Work out the finished part from the listing and answer in its coordinate system (mm). Face numbers are marked on the shaded views. A direction names the side the tool comes from. Round coordinates to 2 decimals unless told otherwise and drop trailing zeros. Write each loop counter-clockwise with the first axis right and the second up, starting at its lowest first coordinate (ties: lowest second). Pieces come first, ordered by that corner, then holes.
Autodesk Inventor part; units mm, degrees
ref_plane "Work Plane1" through (-56.3599, 0, 22) normal (0, 0, -1) x (-1, 0, 0)
ref_plane "YZ Plane" through (0, 0, 0) normal (1, 0, 0) x (0, 1, 0)
ref_plane "XZ Plane" through (0, 0, 0) normal (0, 1, 0) x (-1, 0, 0)
ref_plane "Work Plane1" through (-56.3599, 0, 22) normal (0, 0, -1) x (-1, 0, 0)
sketch "Sketch1" plane through (-56.3599, 0, 22) normal (0, 0, -1) x (-1, 0, 0)
  line L0 (-4.0299, -0.3538) -> (-2.2322, 1.4439) construction
  arc A0 (-1.4439, 2.2322) -> (-2.2322, 1.4439) centre (-0.9299, 0.9299) ccw construction
  line L1 (-1.4439, 2.2322) -> (0.3538, 4.0299) construction
  line L2 (-37.8299, 42.8299) -> (-37.8299, 37.8299) construction
  line L3 (-37.8299, 37.8299) -> (-42.9208, 37.8299) construction
  line L4 (-37.8299, 42.2137) -> (-37.8299, 45.8299) construction
  line L5 (-37.8299, 45.8299) -> (-4.0299, 45.8299) construction
  line L6 (-4.0299, 45.8299) -> (-4.0299, 42.2137) construction
  line L7 (-4.0299, 4.0299) -> (0.3538, 4.0299)
  circle A1 centre (-20.9299, 20.9299) radius 17.5
  line L8 (-20.9299, 58.9723) -> (17.1124, 20.9299) construction
  line L9 (17.1124, 20.9299) -> (-20.9299, -17.1124) construction
  line L10 (-20.9299, -17.1124) -> (-58.9723, 20.9299) construction
  line L11 (-58.9723, 20.9299) -> (-20.9299, 58.9723) construction
  line L12 (-20.9299, 58.9723) -> (-20.9299, -17.1124) construction
  line L13 (17.1124, 20.9299) -> (-58.9723, 20.9299) construction
  line L14 (-20.9299, 58.9723) -> (32.8701, 58.9723) construction
  line L15 (-43.4299, 43.4299) -> (1.5701, 43.4299) construction
  line L16 (1.5701, 43.4299) -> (1.5701, -1.5701) construction
  line L17 (1.5701, -1.5701) -> (-43.4299, -1.5701) construction
  line L18 (-43.4299, -1.5701) -> (-43.4299, 43.4299) construction
  line L19 (-43.4299, 43.4299) -> (1.5701, -1.5701) construction
  line L20 (1.5701, 43.4299) -> (-43.4299, -1.5701) construction
  line L21 (-43.4299, 5.3876) -> (-43.4299, 36.4723)
  line L22 (-43.4299, 36.4723) -> (-36.4723, 43.4299)
  line L23 (-36.4723, 43.4299) -> (-5.3876, 43.4299)
  line L24 (-5.3876, 43.4299) -> (1.5701, 36.4723)
  line L25 (1.5701, 36.4723) -> (1.5701, 5.3876)
  line L26 (1.5701, 5.3876) -> (-5.3876, -1.5701)
  line L27 (-5.3876, -1.5701) -> (-36.4723, -1.5701)
  line L28 (-36.4723, -1.5701) -> (-43.4299, 5.3876)
  line L29 (-4.0299, 42.2137) -> (-37.8299, 42.2137)
  line L30 (-4.0299, -0.3538) -> (-4.0299, 4.0299)
  circle A2 centre (-20.9299, 20.9299) radius 1.5
  line L31 (-10.9299, 10.9299) -> (-30.9299, 10.9299) construction
  line L32 (-30.9299, 10.9299) -> (-30.9299, 30.9299) construction
  line L33 (-30.9299, 30.9299) -> (-10.9299, 30.9299) construction
  line L34 (-10.9299, 30.9299) -> (-10.9299, 10.9299) construction
  line L35 (-10.9299, 10.9299) -> (-30.9299, 30.9299) construction
  line L36 (-30.9299, 10.9299) -> (-10.9299, 30.9299) construction
  circle A3 centre (-30.9299, 30.9299) radius 1.4
  circle A4 centre (-30.9299, 10.9299) radius 1.4
  circle A5 centre (-10.9299, 10.9299) radius 1.4
  line L37 (-45.8299, 37.8299) -> (-42.0723, 37.8299) construction
  line L38 (-42.1723, 37.7299) -> (-45.8299, 37.7299)
  line L39 (-45.8299, 37.7299) -> (-45.8299, 4.1299)
  line L40 (-45.8299, 4.1299) -> (-42.1723, 4.1299)
  line L41 (-42.1723, 4.1299) -> (-42.1723, 37.7299)
  line L42 (-45.8299, 4.0299) -> (-42.0723, 4.0299) construction
  line L43 (-45.8299, 37.8299) -> (-42.0723, 37.8299)
  line L44 (-37.7299, 45.8299) -> (-4.1299, 45.8299)
  line L45 (-4.1299, 45.8299) -> (-4.1299, 42.1723)
  line L46 (-4.1299, 42.1723) -> (-37.7299, 42.1723)
  line L47 (-37.7299, 42.1723) -> (-37.7299, 45.8299)
  line L48 (0.4701, 37.8299) -> (0.4701, 4.0299) construction
  line L49 (0.4701, 4.0299) -> (3.9701, 4.0299) construction
  line L50 (3.9701, 37.8299) -> (3.9701, 4.0299) construction
  line L51 (0.4701, 37.8299) -> (3.9701, 37.8299) construction
  line L52 (-45.8299, -3.9701) -> (-4.0299, -3.9701) construction
  line L53 (0.3124, 37.7299) -> (3.9701, 37.7299)
  line L54 (3.9701, 37.7299) -> (3.9701, 4.1299)
  line L55 (3.9701, 4.1299) -> (0.3124, 4.1299)
  line L56 (0.3124, 4.1299) -> (0.3124, 37.7299)
  line L57 (-4.1713, -0.3538) -> (-37.7299, -0.3538)
  line L58 (-37.7299, -0.3538) -> (-37.7299, -3.9701)
  line L59 (-37.7299, -3.9701) -> (-4.1713, -3.9701)
  line L60 (-4.1713, -3.9701) -> (-4.1713, -0.3538)
  point P0 (-37.8299, 4.0299)
  dimension "d18" = 53.8
  dimension "d19" = 45
  dimension "d20" = 53.8
  dimension "d21" = 45
  dimension "d22" = 45
  dimension "d30" = 20
  dimension "d31" = 20
  dimension "d32" = 2.8
  dimension "d33" = 2.8
  dimension "d34" = 2.8
  dimension "d35" = 3
  dimension "d36" = 0.1
  dimension "d37" = 0.1
  dimension "d38" = 0.1
  dimension "d39" = 0.1
extrude "Extrusion1" add sketch "Sketch1" along normal blind 6 contours L30 L26 L57 L28 L41 L22 L46 L24 L56 L7 | L7 L26 L30 | L56 L24 L25 L26 | L26 L25 L24 L53 L54 L55 | L60 L59 L58 L57 L28 L27 L26 | L26 L27 L28 L57 | L46 L22 L29 L24 | L24 L29 L45 | L40 L39 L38 L22 L21 L28 | L28 L21 L22 L41 | L29 L22 L23 L24 | L24 L23 L22 L29 L47 L44 L45 | L47 L29 L22 | A1 | A2 | A3 | A4 | A5
sketch "Skizze4" plane through (-56.3599, 0, 16) normal (0, 0, -1) x (-1, 0, 0)
  line L0 (-37.7299, 42.1723) -> (-42.1723, 37.7299)
  line L1 (-42.1723, 37.7299) -> (-45.8299, 37.7299)
  line L2 (-45.8299, 37.7299) -> (-45.8299, 4.1299) construction
  line L3 (-45.8299, 4.1299) -> (-42.1723, 4.1299)
  line L4 (-42.1723, 4.1299) -> (-37.6885, -0.3538)
  line L5 (-37.6885, -0.3538) -> (-37.7299, -0.3538)
  line L6 (-37.7299, -0.3538) -> (-37.7299, -3.9701)
  line L7 (-37.7299, -3.9701) -> (-4.1713, -3.9701) construction
  line L8 (-4.1713, -3.9701) -> (-4.1713, -0.3538)
  line L9 (-4.1713, -0.3538) -> (0.3124, 4.1299)
  line L10 (0.3124, 4.1299) -> (3.9701, 4.1299)
  line L11 (3.9701, 4.1299) -> (3.9701, 37.7299) construction
  line L12 (3.9701, 37.7299) -> (0.3124, 37.7299)
  line L13 (0.3124, 37.7299) -> (-4.1299, 42.1723)
  line L14 (-4.1299, 42.1723) -> (-4.1299, 45.8299)
  line L15 (-4.1299, 45.8299) -> (-37.7299, 45.8299) construction
  line L16 (-37.7299, 45.8299) -> (-37.7299, 42.1723)
  line L17 (-37.9299, 46.0299) -> (-3.9299, 46.0299) construction
  line L18 (-3.9299, 46.0299) -> (-3.9299, 42.2551)
  line L19 (-3.9299, 42.2551) -> (0.3953, 37.9299)
  line L20 (0.3953, 37.9299) -> (4.1701, 37.9299)
  line L21 (4.1701, 37.9299) -> (4.1701, 3.9299) construction
  line L22 (4.1701, 3.9299) -> (0.3953, 3.9299)
  line L23 (0.3953, 3.9299) -> (-3.9713, -0.4367)
  line L24 (-3.9713, -0.4367) -> (-3.9713, -4.1701)
  line L25 (-3.9713, -4.1701) -> (-37.9299, -4.1701) construction
  line L26 (-37.9299, -4.1701) -> (-37.9299, -0.3953)
  line L27 (-37.9299, -0.3953) -> (-42.2551, 3.9299)
  line L28 (-42.2551, 3.9299) -> (-46.0299, 3.9299)
  line L29 (-46.0299, 3.9299) -> (-46.0299, 37.9299) construction
  line L30 (-46.0299, 37.9299) -> (-42.2551, 37.9299)
  line L31 (-42.2551, 37.9299) -> (-37.9299, 42.2551)
  line L32 (-37.9299, 42.2551) -> (-37.9299, 46.0299)
  line L33 (-45.8299, 37.7299) -> (-45.8299, 37.9299)
  line L34 (-4.1299, 45.8299) -> (-37.7299, 45.8299)
  line L35 (-37.7299, 45.8299) -> (-37.9299, 45.8299)
  line L36 (-4.1299, 45.8299) -> (-3.9299, 45.8299)
  line L37 (3.9701, 37.7299) -> (3.9701, 37.9299)
  line L38 (3.9701, 4.1299) -> (3.9701, 37.7299)
  line L39 (3.9701, 4.1299) -> (3.9701, 3.9299)
  line L40 (-4.1713, -3.9701) -> (-3.9713, -3.9701)
  line L41 (-37.7299, -3.9701) -> (-37.9299, -3.9701)
  line L42 (-45.8299, 4.1299) -> (-45.8299, 3.9299)
  point P0 (-56.3599, 0)
  dimension "d40" = 0.2
extrude "IM_offset" add sketch "Skizze4" against normal up to surface (6 mm away)
ref_plane "Arbeitsebene5" through (-35.4299, 3.9299, 22) normal (-1, 0, 0) x (0, 0, 1)
ref_plane "Arbeitsebene6" through (-18.4299, 20.9299, 22) normal (0, 1, 0) x (-1, 0, 0)
sketch "Skizze31" plane through (-56.3599, 0, 16) normal (0, 0, -1) x (-1, 0, 0)
  line L0 (3.9701, 3.9299) -> (3.9701, 37.9299)
  line L1 (3.9701, 37.9299) -> (0.3953, 37.9299)
  line L2 (0.3953, 37.9299) -> (-3.9299, 42.2551)
  line L3 (-3.9299, 42.2551) -> (-3.9299, 45.8299)
  line L4 (-3.9299, 45.8299) -> (-37.9299, 45.8299)
  line L5 (-37.9299, 45.8299) -> (-37.9299, 42.2551)
  line L6 (-37.9299, 42.2551) -> (-42.2551, 37.9299)
  line L7 (-42.2551, 37.9299) -> (-45.8299, 37.9299)
  line L8 (-45.8299, 37.9299) -> (-45.8299, 3.9299)
  line L9 (-42.2551, 3.9299) -> (-45.8299, 3.9299)
  line L10 (-37.9299, -0.3953) -> (-42.2551, 3.9299)
  line L11 (-37.9299, -3.9701) -> (-37.9299, -0.3953)
  line L12 (-3.9713, -3.9701) -> (-37.9299, -3.9701)
  line L13 (-3.9713, -3.9701) -> (-3.9713, -0.4367)
  line L14 (-3.9713, -0.4367) -> (0.3953, 3.9299)
  line L15 (0.3953, 3.9299) -> (3.9701, 3.9299)
  circle A0 centre (-20.9506, 20.9092) radius 10
  point P0 (-56.3599, 0)
  dimension "d181" = 20
extrude "Extrusion26" cut sketch "Skizze31" against normal blind 10 contours A0
sketch "Skizze32" plane through (-56.3599, 0, 16) normal (0, 0, -1) x (-1, 0, 0)
  circle A0 centre (-20.9506, 20.9092) radius 10
  circle A1 centre (-20.9506, 20.9092) radius 15
  line L0 (-3.6301, 10.9092) -> (-38.2711, 10.9092)
  line L1 (-38.2711, 10.9092) -> (-20.9506, 40.9092)
  line L2 (-20.9506, 40.9092) -> (-3.6301, 10.9092)
  line L3 (-3.9713, -3.9701) -> (-37.9299, -3.9701)
  circle A2 centre (-3.6301, 10.9092) radius 2.5
  circle A3 centre (-38.2711, 10.9092) radius 2.5
  circle A4 centre (-20.9506, 40.9092) radius 2.5
  circle A5 centre (-3.6301, 10.9092) radius 4 construction
  circle A6 centre (-38.2711, 10.9092) radius 4 construction
  circle A7 centre (-20.9506, 40.9092) radius 4 construction
  point P0 (-56.3599, 0)
  dimension "d184" = 30
  dimension "d185" = 10
  dimension "d186" = 5
  dimension "d187" = 5
  dimension "d188" = 5
  dimension "d189" = 8
  dimension "d190" = 8
  dimension "d191" = 8
extrude "Extrusion27" add sketch "Skizze32" along normal blind 4 contours A4 L1 L2 | L2 L1 A4 | A2 L0 L2 | L2 L0 A2 | A3 L1 L0 | L0 L1 A3
sketch "Skizze33" plane through (-56.3599, 0, 16) normal (0, 0, -1) x (-1, 0, 0)
  circle A0 centre (-38.2711, 10.9092) radius 2.5
  circle A1 centre (-3.6301, 10.9092) radius 2.5
  circle A2 centre (-20.9506, 40.9092) radius 2.5
  circle A3 centre (-20.9506, 20.9092) radius 10
  line L0 (3.9701, 3.9299) -> (3.9701, 37.9299)
  line L1 (3.9701, 37.9299) -> (0.3953, 37.9299)
  line L2 (0.3953, 37.9299) -> (-3.9299, 42.2551)
  line L3 (-3.9299, 42.2551) -> (-3.9299, 45.8299)
  line L4 (-3.9299, 45.8299) -> (-37.9299, 45.8299)
  line L5 (-37.9299, 45.8299) -> (-37.9299, 42.2551)
  line L6 (-37.9299, 42.2551) -> (-42.2551, 37.9299)
  line L7 (-42.2551, 37.9299) -> (-45.8299, 37.9299)
  line L8 (-45.8299, 37.9299) -> (-45.8299, 3.9299)
  line L9 (-42.2551, 3.9299) -> (-45.8299, 3.9299)
  line L10 (-37.9299, -0.3953) -> (-42.2551, 3.9299)
  line L11 (-37.9299, -3.9701) -> (-37.9299, -0.3953)
  line L12 (-3.9713, -3.9701) -> (-37.9299, -3.9701)
  line L13 (-3.9713, -3.9701) -> (-3.9713, -0.4367)
  line L14 (-3.9713, -0.4367) -> (0.3953, 3.9299)
  line L15 (0.3953, 3.9299) -> (3.9701, 3.9299)
  circle A4 centre (-20.9506, 40.9092) radius 3
  circle A5 centre (-3.6301, 10.9092) radius 3
  circle A6 centre (-38.2711, 10.9092) radius 3
  point P0 (-56.3599, 0)
  dimension "d194" = 0.5
  dimension "d195" = 0.5
  dimension "d196" = 0.5
extrude "Extrusion28" add sketch "Skizze33" along normal blind 1 contours A0 | A1 | A4 | A5 | A6
properties part number "20_Cube_Insert_rotational_filtermount_v3.iam"
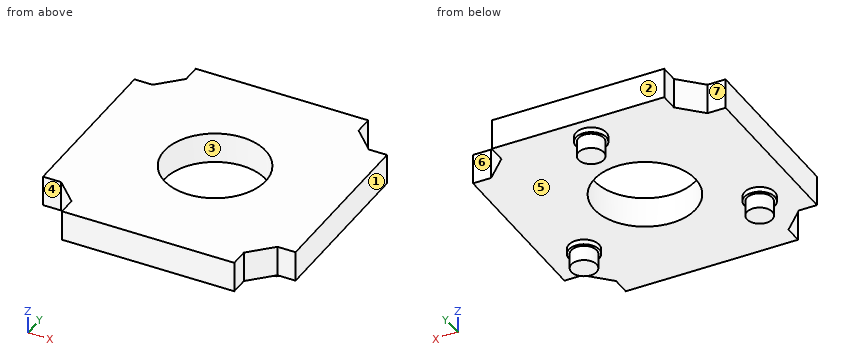
Q1. Find section C-C (z = 18.25). Determine the outline of the cut face in (x, y).
Q2. Find section A-A (y = 25). Determine the outline of the cut face in (x, z), plus the area to 3 significant figures.
Q3. Find section B-B (x = -41). Determine the outline of the cut face in (y, z).
Q4. The mould has two halves that part along Y. Classify the marked faces 1, 2 and 3: +Y half, -Y half, draft (parallel to the pull), parting line (faces both ways), or undercut.
Q5. Given pin 1 (1.8 mm diameter, centred on x = -58.5, z = 18.5, fed in from -Y); pin 2 (3 mm diameter, centred on y = -3, z = 19.5, fed in from +X); pin 3 (1.5 mm diameter, centred on y = 32, z = 14.5, fed in from -X); pin 4 (12 mm diameter, centred on x = -23.5, y = 39, fed in from -Z), each flat-ended and moving along its own axis, determine where each tip first touches the part or whether it passes through.
Q6. Find section D-D (y = 11.5). Determine the outline of the cut face in (x, z).
Q7. A tool of negligible diameter and unlimited length cuts with its end or side. For the marked faces 4, 5, 6 and 7, from which of +Z, -Z, +X, -X, +Y, -Y can it reach the whole face along a straight path? Write none if from no direction.
Q8. Find the intervals of material crossed by L1, parallel to Z at x = -44.5, y = 41; L2, parallel to X at y = 44, z = 18.75; L3, parallel to X at y = 27, z = 19.25, in increasing order.
Report:
1. outline: (-60.33, 3.93) - (-56.76, 3.93) - (-52.39, -0.44) - (-52.39, -3.97) - (-18.43, -3.97) - (-18.43, -0.4) - (-14.1, 3.93) - (-10.53, 3.93) - (-10.53, 37.93) - (-14.1, 37.93) - (-18.43, 42.26) - (-18.43, 45.83) - (-52.43, 45.83) - (-52.43, 42.26) - (-56.76, 37.93) - (-60.33, 37.93) - close; hole circle Ø20 at (-35.41, 20.91)
2. outline: (-60.33, 16) - (-44.53, 16) - (-44.53, 22) - (-60.33, 22) - close; (-26.28, 16) - (-10.53, 16) - (-10.53, 22) - (-26.28, 22) - close
2. area: 189 mm2
3. outline: (-3.97, 16) - (12.62, 16) - (12.62, 22) - (-3.97, 22) - close; (29.2, 16) - (45.83, 16) - (45.83, 22) - (29.2, 22) - close
4. face 1: draft
4. face 2: +Y half
4. face 3: undercut
5. pin 1: stops at y = 3.93
5. pin 2: stops at x = -18.43
5. pin 3: passes through
5. pin 4: stops at z = 16
6. outline: (-60.33, 16) - (-55.67, 16) - (-55.67, 15) - (-55.16, 15) - (-55.16, 12) - (-50.3, 12) - (-50.3, 15) - (-49.79, 15) - (-49.79, 16) - (-38.8, 16) - (-38.8, 22) - (-60.33, 22) - close; (-32.02, 16) - (-21.03, 16) - (-21.03, 15) - (-20.52, 15) - (-20.52, 12) - (-15.66, 12) - (-15.66, 15) - (-15.15, 15) - (-15.15, 16) - (-10.53, 16) - (-10.53, 22) - (-32.02, 22) - close
7. face 4: +Z, -Z, -X, -Y
7. face 5: -Z
7. face 6: +Z, -Z, +X, +Y
7. face 7: +Z, -Z, -X, +Y
8. L1: z = 16 to 22
8. L2: x = -52.43 to -18.43
8. L3: x = -60.33 to -43.34, -27.48 to -10.53
